```python
from build123d import *

# Parameters (mm, degrees)
SKETCH_1_W               = 47
SKETCH_1_H               = 5
EXTRUDE_1_DEPTH          = 19
SKETCH_2_R               = 23.5
EXTRUDE_2_DEPTH          = 5
M2_5X0_45_1_D            = 2.05
M2_5X0_45_1_DEPTH        = 7.25
M2_5X0_45_1_TIP          = 0.615882135
CUT_EXTRUDE_1_DEPTH      = 5
CUT_EXTRUDE_2_DEPTH      = 1
CUT_EXTRUDE_2_DEPTH_BACK = 6
CUT_EXTRUDE_3_DEPTH      = 5


with BuildPart() as part:
    # ｽｹｯﾁ1 → ﾎﾞｽ - 押し出し1 (new body)
    with BuildSketch(Plane.XY):
        Rectangle(SKETCH_1_W, SKETCH_1_H)
    extrude(amount=EXTRUDE_1_DEPTH)

    # ｽｹｯﾁ2 → ﾎﾞｽ - 押し出し2 (add)
    with BuildSketch(Plane.XZ.offset(2.5)):
        with Locations((0, 19)):
            Circle(SKETCH_2_R)
    extrude(amount=-EXTRUDE_2_DEPTH)

    # M2.5x0.45 ねじ穴1
    with Locations(Plane(origin=(0, 0, 0), x_dir=(-1, 0, 0), z_dir=(0, 0, -1))):
        with Locations((18, 0), (-18, 0)):
            Hole(M2_5X0_45_1_D / 2, depth=M2_5X0_45_1_DEPTH)
            with Locations((0, 0, -(M2_5X0_45_1_DEPTH + M2_5X0_45_1_TIP / 2))):  # 118° drill point
                Cone(0, M2_5X0_45_1_D / 2, M2_5X0_45_1_TIP, mode=Mode.SUBTRACT)

    # ｽｹｯﾁ3 → ｶｯﾄ - 押し出し1 (cut)
    with BuildSketch(Plane.XZ.offset(2.5)):
        with BuildLine():
            Line((14, 19), (0, 19))
            Line((0, 19), (-14, 19))
            ThreePointArc((-14, 19), (0, 5), (14, 19))
        make_face()
        with BuildLine():
            Line((-14, 19), (0, 19))
            Line((0, 19), (14, 19))
            ThreePointArc((14, 19), (0, 33), (-14, 19))
        make_face()
    extrude(amount=-CUT_EXTRUDE_1_DEPTH, mode=Mode.SUBTRACT)

    # ｽｹｯﾁ10 → ｶｯﾄ - 押し出し2 (cut, two sides)
    with BuildSketch(Plane.XZ.offset(2.5)) as cut_extrude_2_sk:
        Polygon((136.961591201, 0), (13.829316686, 0), (-13.829316686, 0), (-136.961591201, 0), (-136.961591201, -246.26454903), (136.961591201, -246.26454903), align=None)
    extrude(amount=CUT_EXTRUDE_2_DEPTH, mode=Mode.SUBTRACT)
    extrude(cut_extrude_2_sk.sketch, amount=-CUT_EXTRUDE_2_DEPTH_BACK, mode=Mode.SUBTRACT)

    # ｽｹｯﾁ11 → ｶｯﾄ - 押し出し3 (cut)
    with BuildSketch(Plane(origin=(0, 2.5, 0), x_dir=(1, 0, 0), z_dir=(0, 1, 0))):
        with BuildLine():
            Line((-10, -40.266170318), (10, -40.266170318))
            ThreePointArc((10, -40.266170318), (0, -42.5), (-10, -40.266170318))
        make_face()
    extrude(amount=-CUT_EXTRUDE_3_DEPTH, mode=Mode.SUBTRACT)


solid = part.part
```
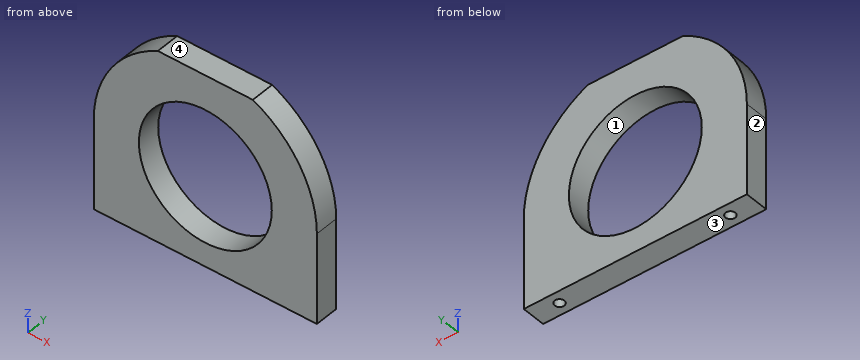
Model file for the job. Use its own axes, mm. Face numbers are marked on the shaded views. Round coordinates to 2 decimals unless told otherwise and drop trailing zeros. Write each loop counter-clockwise with the first axis right and the second up, starting at its lowest first coordinate (ties: lowest second). Pieces come first, ordered by that corner, then holes. Notation, with made-up numbers: (75, 44) - (84, 44) arc R14 cw to (84, 59) - close; hole circle Ø6 at (42.5, 22). An arc over 180 degrees is marked (long way). One line per item, written item: value.
(1) Wall check: probe 1 along Y at (x, z) = (18, 4) (3 decimals); probe 2 along Z at (x, y) = (0, -0.45); probe 3 along X at (y, z) = (1.65, 19.5). Give the ranges that are in metal, low to high.
Values follow:
probe 1: y = -2.5 to -1.025, 1.025 to 2.5
probe 2: z = 0 to 5, 33 to 40.27
probe 3: x = -23.49 to -13.99, 13.99 to 23.49
(2) Cut at B-B, the plane x = 0. Give the cut face in (y, z).
Values follow:
outline: (-2.5, 0) - (2.5, 0) - (2.5, 5) - (-2.5, 5) - close; (-2.5, 33) - (2.5, 33) - (2.5, 40.27) - (-2.5, 40.27) - close
(3) Two-plate mould, pull along Z, no slides. Class the marked faces 1, 2, 3 and 4: pulls with the +Z half, pulls with the -Z half, needs draft (parallel to the pull), parting line crosses it, or undercut.
Values follow:
face 1: undercut
face 2: needs draft
face 3: pulls with the -Z half
face 4: pulls with the +Z half
(4) Cut at A-A, the plane y = -1.8. Give the cut face in (x, z), plus the area to 3 significant figures.
Values follow:
outline: (-23.5, 0) - (23.5, 0) - (23.5, 19) arc R23.5 ccw to (10, 40.27) - (-10, 40.27) arc R23.5 ccw to (-23.5, 19) - close; hole circle Ø28 at (0, 19)
area: 1,110 mm²
(5) Cut at C-C, the plane z = 22.5. Give the cut face in (x, y).
Values follow:
outline: (-23.24, -2.5) - (-13.56, -2.5) - (-13.56, 2.5) - (-23.24, 2.5) - close; (13.56, -2.5) - (23.24, -2.5) - (23.24, 2.5) - (13.56, 2.5) - close
(6) Drop flat-ended pins along their axis: P1, Ø2.5, axis at x = 18, y = 0, coming from the +Z side; P2, Ø8, axis at x = 3, z = 5.5, coming from the -Y side; P3, Ø3, axis at y = 0, z = 31, coming from the -X side. Give the stop position or say it passes through.
Values follow:
P1: stops at z = 35.48
P2: stops at y = -2.5
P3: stops at x = -21.02
